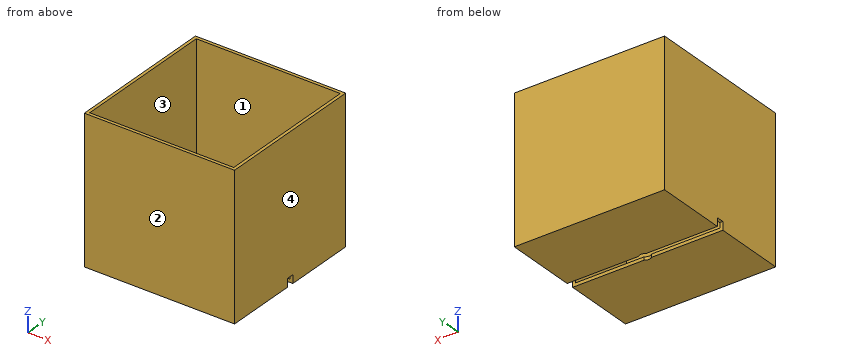
```python
from build123d import *

# Parameters (mm, degrees)
F0_W     = 73
F0_H     = 73
F1_DEPTH = 70
F2_T     = -1.5
F4_DEPTH = 4


with BuildPart() as f1:
    # F0 (on Top) → F1 (new body)
    with BuildSketch(Plane.XY):
        Rectangle(F0_W, F0_H)
    extrude(amount=F1_DEPTH)

    # F2
    f2_openings = [f1.faces().sort_by_distance(p)[0] for p in [
        (0, 0, 70),
    ]]
    offset(amount=F2_T, openings=f2_openings)

    # F3 (on face) → F4 (cut)
    with BuildSketch(Plane(origin=(0, 0, 0), x_dir=(1, 0, 0), z_dir=(0, 0, -1))):
        with BuildLine():
            Line((1.7349351573, -1.8), (36.5, -1.8))
            Line((36.5, -1.8), (36.5, 1.8))
            Line((36.5, 1.8), (1.7349351573, 1.8))
            ThreePointArc((1.7349351573, 1.8), (2.3007974588, 0.9779218033), (2.5, 0))
            ThreePointArc((2.5, 0), (2.3007974588, -0.9779218033), (1.7349351573, -1.8))
        make_face()
        with BuildLine():
            ThreePointArc((-1.7349351573, -1.8), (0, -2.5), (1.7349351573, -1.8))
            Line((1.7349351573, -1.8), (-1.7349351573, -1.8))
        make_face()
        with BuildLine():
            Line((-1.7349351573, -1.8), (1.7349351573, -1.8))
            ThreePointArc((1.7349351573, -1.8), (2.3007974588, -0.9779218033), (2.5, 0))
            ThreePointArc((2.5, 0), (2.3007974588, 0.9779218033), (1.7349351573, 1.8))
            Line((1.7349351573, 1.8), (-1.7349351573, 1.8))
            ThreePointArc((-1.7349351573, 1.8), (-2.5, 0), (-1.7349351573, -1.8))
        make_face()
        with BuildLine():
            Line((-36.5, -1.8), (-1.7349351573, -1.8))
            ThreePointArc((-1.7349351573, -1.8), (-2.5, 0), (-1.7349351573, 1.8))
            Line((-1.7349351573, 1.8), (-36.5, 1.8))
            Line((-36.5, 1.8), (-36.5, -1.8))
        make_face()
        with BuildLine():
            Line((-1.7349351573, 1.8), (1.7349351573, 1.8))
            ThreePointArc((1.7349351573, 1.8), (0, 2.5), (-1.7349351573, 1.8))
        make_face()
    extrude(amount=-F4_DEPTH, mode=Mode.SUBTRACT)


solid = f1.part
```
Design review of the part built by this model. Coordinates are the model's own, in mm. Face numbers are marked on the shaded views. Coordinates: 2 decimals unless noted, no trailing zeros. Order: outer loops, then holes, each group sorted by start corner. A loop starts at its lowest first (then second) coordinate and runs counter-clockwise, first axis right, second up. Notation, with made-up numbers: M 30,44.25 L 38,44.25 A19 ccw 38,69.25 Z; hole C 38,25.25 d9. An arc over 180 degrees is marked long. Answer as a JSON object with one key per item and string values. Group by question number.
1) Add section B-B, the plane z = 30. Write out the cut boundary in (x, y).
2) Mouldability with a two-part tool opening along Y and no side actions: class the marked faces 1, 2, 3 and 4 as pulls with the +Y half, pulls with the -Y half, needs draft (parallel to the pull), parting line crosses it, or undercut.
3) For pin 1 (5 mm diameter, centred on x = 25.5, y = -0.5, fed in from +Z); pin 2 (1.2 mm diameter, centred on x = -36, y = 0, fed in from -Z), all flat-tipped, find the tip position at first contact; note any pin that passes through.
4) Add section A-A, the plane x = -23. Write out the cut boundary in (y, z), then the cut area to 3 significant figures.
5) Add section C-C, the plane y = 21. Write out the cut boundary in (x, z), then the cut area to 3 significant figures.
6) Wall thickness on L1, parallel to Y at x = 0, z = 36; L2, parallel to Z at x = -0.5, y = -20: over which ranges is each line inside the solid? List them lowest first.
Computed values:
{
 "1": {"outline": "M -36.5,-36.5 L 36.5,-36.5 L 36.5,36.5 L -36.5,36.5 Z; hole M -35,-35 L 35,-35 L 35,35 L -35,35 Z"},
 "2": {"face 1": "undercut", "face 2": "pulls with the -Y half", "face 3": "undercut", "face 4": "needs draft"},
 "3": {"pin 1": "stops at z = 1.5", "pin 2": "stops at z = 4"},
 "4": {"outline": "M -36.5,0 L -1.8,0 L -1.8,1.5 L -35,1.5 L -35,70 L -36.5,70 Z; M 1.8,0 L 36.5,0 L 36.5,70 L 35,70 L 35,1.5 L 1.8,1.5 Z", "area": "310 mm^2"},
 "5": {"outline": "M -36.5,0 L 36.5,0 L 36.5,70 L 35,70 L 35,1.5 L -35,1.5 L -35,70 L -36.5,70 Z", "area": "315 mm^2"},
 "6": {"L1": "y = -36.5 to -35, 35 to 36.5", "L2": "z = 0 to 1.5"}
}
